Design review of the part built by this model. Coordinates are the model's own, in mm. A direction names the side the tool comes from. Give positions to 0.01 mm unless a question says otherwise; leave off trailing zeros. Loops run counter-clockwise (first coordinate to the right, second up) from the corner with the lowest first, then second, coordinate; pieces in that order, holes last. Notation, with made-up numbers: M -12,-14 L 0,-14 A27 cw 0,14 Z; hole C 86.25,-5.75 d8. An arc over 180 degrees is marked long. Use a Markdown table: item, result. Add a question column.
(1) For faces 5 (the face through (1.016, 3, 1)), 6 (the face through (2.76, 6.76, 10.47)), 7 (the face through (5, 3, 13.716)), 8 (the face through (4, 0, 7)), list the 3-axis set-ups (+Z, -Z, +X, -X, +Y, -Y) from which the entire face can be reached by the end or side of a thin tool; tool diameter is ignored.
(2) Draft analysis for pull direction Y (two halves, no side actions). For faces 1 (the face through (4, 5, 14.224)), 2 (the face through (6.803, 7.602, 7.012)), 3 (the face through (5, 0.508, 12)), 4 (the face through (5.3, 4.572, 12.2)), state which applies: pulls with the +Y half, pulls with the -Y half, needs draft (parallel to the pull), parting line crosses it, or undercut.
(3) Add section A-A, the plane x = 5.5. Give the boundary of the cut face in (y, z).
(4) Add section B-B, the plane z = 2.54. Give the boundary of the cut face in (x, y), then the cut area to 3 significant figures.
(5) Insertion check: pin 1 Ø1.2 at (y, z) = (2, 3.5) entering from +X; pin 2 Ø2 at (x, z) = (4.5, 3) entering from -Y. Each pin has a flat end and moves straight along its axis. Give the tip position at first contact, or say it passes through.
(6) Add section C-C, the plane y = 3.5. Give the boundary of the cut face in (x, z), then the cut area to 3 significant figures.
(7) Add section D-D, the plane y = 6. Give the boundary of the cut face in (x, z), then the cut area to 3 significant figures.
(8) For probe 1 along Z at (x, y) = (3.25, 1.75); probe 2 along Y at (x, z) = (4.25, 4); probe 3 along X at (y, z) = (5.25, 7), list the stretches that pass through material, from the lowest coordinate up.
```python
from build123d import *

# Parameters (mm, degrees)
EXTRUDE_1_DEPTH     = 14.224
SKETCH_2_R          = 1.524
CUT_EXTRUDE_1_DEPTH = 8.382
SKETCH_3_W          = 4.064
SKETCH_3_H          = 4.064
CUT_EXTRUDE_2_DEPTH = 5.334
SKETCH_4_W          = 0.762
SKETCH_4_H          = 6.35
CUT_EXTRUDE_3_DEPTH = 1.27


with BuildPart() as part:
    # 草图1 → 凸台-拉伸1 (new body)
    with BuildSketch(Plane.XY):
        Polygon((0, 0), (7.366, 0), (7.366, 6.35), (6.223, 8.89), (1.143, 8.89), (0, 6.35), align=None)
    extrude(amount=EXTRUDE_1_DEPTH)

    # 草图2 → 切除-拉伸1 (cut)
    with BuildSketch(Plane(origin=(0, 8.89, 0), x_dir=(1, 0, 0), z_dir=(0, 1, 0))):
        with Locations(Location((3.683, -2.54, 0), (0, 0, 270))):
            Circle(SKETCH_2_R)
        with Locations(Location((3.683, -11.684, 0), (0, 0, 270))):
            Circle(SKETCH_2_R)
        with Locations(Location((3.683, -7.112, 0), (0, 0, 270))):
            Circle(SKETCH_2_R)
    extrude(amount=-CUT_EXTRUDE_1_DEPTH, mode=Mode.SUBTRACT)

    # 草图3 → 切除-拉伸2 (cut)
    with BuildSketch(Plane(origin=(7.366, 0, 0), x_dir=(0, 0, -1), z_dir=(1, 0, 0))):
        with Locations((-11.684, 2.54)):
            Rectangle(SKETCH_3_W, SKETCH_3_H)
        Polygon((-7.112, 0.508), (-9.144, 0.508), (-9.144, 4.572), (-5.08, 4.572), (-5.08, 0.508), align=None)
        with Locations((-2.54, 2.54)):
            Rectangle(SKETCH_3_W, SKETCH_3_H)
    extrude(amount=-CUT_EXTRUDE_2_DEPTH, mode=Mode.SUBTRACT)

    # 草图4 → 切除-拉伸3 (cut)
    with BuildSketch(Plane.XY):
        with Locations((1.397, 3.175)):
            Rectangle(SKETCH_4_W, SKETCH_4_H)
    extrude(amount=CUT_EXTRUDE_3_DEPTH, mode=Mode.SUBTRACT)


solid = part.part
```
Established:
| question | item | result |
|---|---|---|
| 1 | face 5 | -Z, -Y |
| 1 | face 6 | +Y |
| 1 | face 7 | +X |
| 1 | face 8 | +Z, -Z, +X, -X, -Y |
| 2 | face 1 | needs draft |
| 2 | face 2 | pulls with the +Y half |
| 2 | face 3 | undercut |
| 2 | face 4 | undercut |
| 3 | outline | M 0,0 L 8.89,0 L 8.89,14.22 L 0,14.22 Z; hole M 0.51,0.51 L 4.57,0.51 L 4.57,4.57 L 0.51,4.57 Z; hole M 0.51,5.08 L 4.57,5.08 L 4.57,9.14 L 0.51,9.14 Z; hole M 0.51,9.65 L 4.57,9.65 L 4.57,13.72 L 0.51,13.72 Z |
| 4 | outline | M 0,0 L 7.37,0 L 7.37,0.51 L 2.03,0.51 L 2.03,4.57 L 2.16,4.57 L 2.16,8.89 L 1.14,8.89 L 0,6.35 Z; M 5.21,4.57 L 7.37,4.57 L 7.37,6.35 L 6.22,8.89 L 5.21,8.89 Z |
| 4 | area | 27.7 mm^2 |
| 5 | pin 1 | x = 2.03 |
| 5 | pin 2 | y = 0 |
| 6 | outline | M 0,0 L 1.02,0 L 1.02,1.27 L 1.78,1.27 L 1.78,0 L 7.37,0 L 7.37,0.51 L 2.03,0.51 L 2.03,4.57 L 7.37,4.57 L 7.37,5.08 L 2.03,5.08 L 2.03,9.14 L 7.37,9.14 L 7.37,9.65 L 2.03,9.65 L 2.03,13.72 L 7.37,13.72 L 7.37,14.22 L 0,14.22 Z |
| 6 | area | 38.8 mm^2 |
| 7 | outline | M 0,0 L 1.02,0 L 1.02,1.27 L 1.78,1.27 L 1.78,0 L 7.37,0 L 7.37,14.22 L 0,14.22 Z; hole C 3.68,2.54 d3.05; hole C 3.68,7.11 d3.05; hole C 3.68,11.68 d3.05 |
| 7 | area | 81.9 mm^2 |
| 8 | probe 1 | 0 to 0.51, 4.57 to 5.08, 9.14 to 9.65, 13.72 to 14.22 |
| 8 | probe 2 | 0 to 0.51, 4.57 to 8.89 |
| 8 | probe 3 | 0 to 2.16, 5.2 to 7.37 |
